Source: CAD feature listing. Evaluate the final solid. Frame: model axes, mm. A direction names the side the tool comes from. Round coordinates to 2 decimals unless told otherwise and drop trailing zeros. Loops run counter-clockwise (first coordinate to the right, second up) from the corner with the lowest first, then second, coordinate; pieces in that order, holes last. Notation, with made-up numbers: M -31,17 L -1,17 A35 cw -1,54 Z; hole C 34,52 d10. An arc over 180 degrees is marked long. One line per item, written item: value.
from build123d import *

# Parameters (mm, degrees)
F0_W      = 67
F0_H      = 50
F1_DEPTH  = 70
F3_DEPTH  = 1.5
F4_W      = 58
F4_H      = 3.3
F5_DEPTH  = 67.001
F6_DEPTH  = 67.001
F7_R      = 3.15
F8_DEPTH  = 12.5
F11_R     = 20
F12_DEPTH = 1.5
F13_R     = 20
F14_DEPTH = 1.5


with BuildPart() as f1:
    # F0 (on Top) → F1 (new body)
    with BuildSketch(Plane.XY):
        Rectangle(F0_W, F0_H)
    extrude(amount=F1_DEPTH)

    # F2 (on face) → F3 (cut)
    with BuildSketch(Plane.XZ.offset(25)):
        Polygon((0, 41.941864), (-26.855644, 70), (-33.5, 70), (-33.5, 63.058136), (-6.644356, 35), (-33.5, 6.941864), (-33.5, 0), (-26.855644, 0), (0, 28.058136), (26.855644, 0), (33.5, 0), (33.5, 6.941864), (6.644356, 35), (33.5, 63.058136), (33.5, 70), (26.855644, 70), align=None)
    extrude(amount=-F3_DEPTH, mode=Mode.SUBTRACT)

    # F4 (on face) → F5 (cut, through all)
    with BuildSketch(Plane.YZ.offset(33.5)):
        with BuildLine():
            Line((33.286914, 36.5), (18.454483, 36.5))
            ThreePointArc((18.454483, 36.5), (-17, 27), (18.454483, 17.5))
            Line((18.454483, 17.5), (33.286914, 17.5))
            Line((33.286914, 17.5), (33.286914, 36.5))
        make_face()
        with Locations((25, 55.85)):
            Rectangle(F4_W, F4_H)
    extrude(amount=-F5_DEPTH, mode=Mode.SUBTRACT)

    # F4 (on face) → F6 (cut, through all)
    with BuildSketch(Plane.YZ.offset(33.5)):
        with BuildLine():
            Line((33.286914, 36.5), (18.454483, 36.5))
            ThreePointArc((18.454483, 36.5), (-17, 27), (18.454483, 17.5))
            Line((18.454483, 17.5), (33.286914, 17.5))
            Line((33.286914, 17.5), (33.286914, 36.5))
        make_face()
        with Locations((25, 55.85)):
            Rectangle(F4_W, F4_H)
    extrude(amount=-F6_DEPTH, mode=Mode.SUBTRACT)

    # F7 (on face) → F8 (cut, through all)
    with BuildSketch(Plane.XY.offset(70)):
        with Locations((0, 16.7)):
            Circle(F7_R)
    extrude(amount=-F8_DEPTH, mode=Mode.SUBTRACT)

    # F11 (on offset) → F12 (cut)
    with BuildSketch(Plane.YZ.offset(21)):
        with Locations((2, 27)):
            Circle(F11_R)
    extrude(amount=-F12_DEPTH, mode=Mode.SUBTRACT)

    # F13 (on offset) → F14 (cut)
    with BuildSketch(Plane.YZ.offset(-21)):
        with Locations((2, 27)):
            Circle(F13_R)
    extrude(amount=F14_DEPTH, mode=Mode.SUBTRACT)


solid = f1.part
1. Pull-direction query (Y, two-part tool) for faces 1 (the face through (0.273, -16.987, 27.696)), 2 (the face through (13.24, -24.26, 14.225)), 3 (the face through (0, 25, 9)); classes: released by +Y, released by -Y, zero draft, split by the parting line, or undercut.
Report:
face 1: undercut
face 2: zero draft
face 3: released by +Y
2. Ray query, line 1 (X direction, y = -12, z = 41); line 2 (Z direction, x = -20.1, y = 2); line 3 (Z direction, x = -17, y = 23). Return the intervals inside material, ascending. Write a range as [from, to].
Report:
line 1: x = [-33.5, -21], [-19.5, 19.5], [21, 33.5]
line 2: z = [0, 7], [47, 54.2], [57.5, 70]
line 3: z = [0, 17.5], [36.5, 54.2], [57.5, 70]
3. Reachability of faces 4 (the face through (-21, -17.4, 27.1)), 5 (the face through (19.88, -24.26, 48.83)), 6 (the face through (0, 25, 64)), 7 (the face through (0, 22, 36.5)) from +Z, -Z, +X, -X, +Y, -Y: full face, straight path, thin tool, end or side. Return the list, or none.
Report:
face 4: none
face 5: -Y
face 6: +Z, -Z, +X, -X, +Y
face 7: +X, -X, +Y
4. Section query D-D (y = -13). Return the cut outline in (x, z), and give its area (3 significant figures).
Report:
outline: M -33.5,0 L 33.5,0 L 33.5,15.34 L 21,15.34 L 21,13.77 L 19.5,13.77 L 19.5,15.34 L -19.5,15.34 L -19.5,13.77 L -21,13.77 L -21,15.34 L -33.5,15.34 Z; M -33.5,38.66 L -21,38.66 L -21,40.23 L -19.5,40.23 L -19.5,38.66 L 19.5,38.66 L 19.5,40.23 L 21,40.23 L 21,38.66 L 33.5,38.66 L 33.5,70 L -33.5,70 Z
area: 3,120 mm2
5. Pin query (flat end, axial travel): pin 1 (2 mm diameter, centred on x = 10.5, z = 19.5, fed in from -Y); pin 2 (19 mm diameter, centred on y = 0, z = 24.5, fed in from +X); pin 3 (12 mm diameter, centred on x = 13.5, z = 27, fed in from -Y); pin 4 (1.6 mm diameter, centred on x = 6.5, z = 56.5, fed in from +Y). Return the tip coordinate at first contact, or that it passes through.
Report:
pin 1: stops at y = -23.5
pin 2: passes through
pin 3: stops at y = -25
pin 4: stops at y = -4
6. Section query A-A (y = 2). Return the cut outline in (x, z).
Report:
outline: M -33.5,0 L 33.5,0 L 33.5,8 L 21,8 L 21,7 L 19.5,7 L 19.5,8 L -19.5,8 L -19.5,7 L -21,7 L -21,8 L -33.5,8 Z; M -33.5,46 L -21,46 L -21,47 L -19.5,47 L -19.5,46 L 19.5,46 L 19.5,47 L 21,47 L 21,46 L 33.5,46 L 33.5,54.2 L -33.5,54.2 Z; M -33.5,57.5 L 33.5,57.5 L 33.5,70 L -33.5,70 Z
7. Section query C-C (x = -2). Return the cut outline in (y, z).
Report:
outline: M -25,0 L 25,0 L 25,17.5 L 18.45,17.5 A19 cw long 18.45,36.5 L 25,36.5 L 25,54.2 L -4,54.2 L -4,57.5 L 14.27,57.5 L 14.27,70 L -25,70 L -25,44.03 L -23.5,44.03 L -23.5,25.97 L -25,25.97 Z; M 19.13,57.5 L 25,57.5 L 25,70 L 19.13,70 Z
8. Section query B-B (y = 16.7). Count the separate pieces of the cut face and the enclosed holes in it, and give its area (3 significant figures).
Report:
separate pieces: 4
enclosed holes: 0
area: 2,770 mm2
